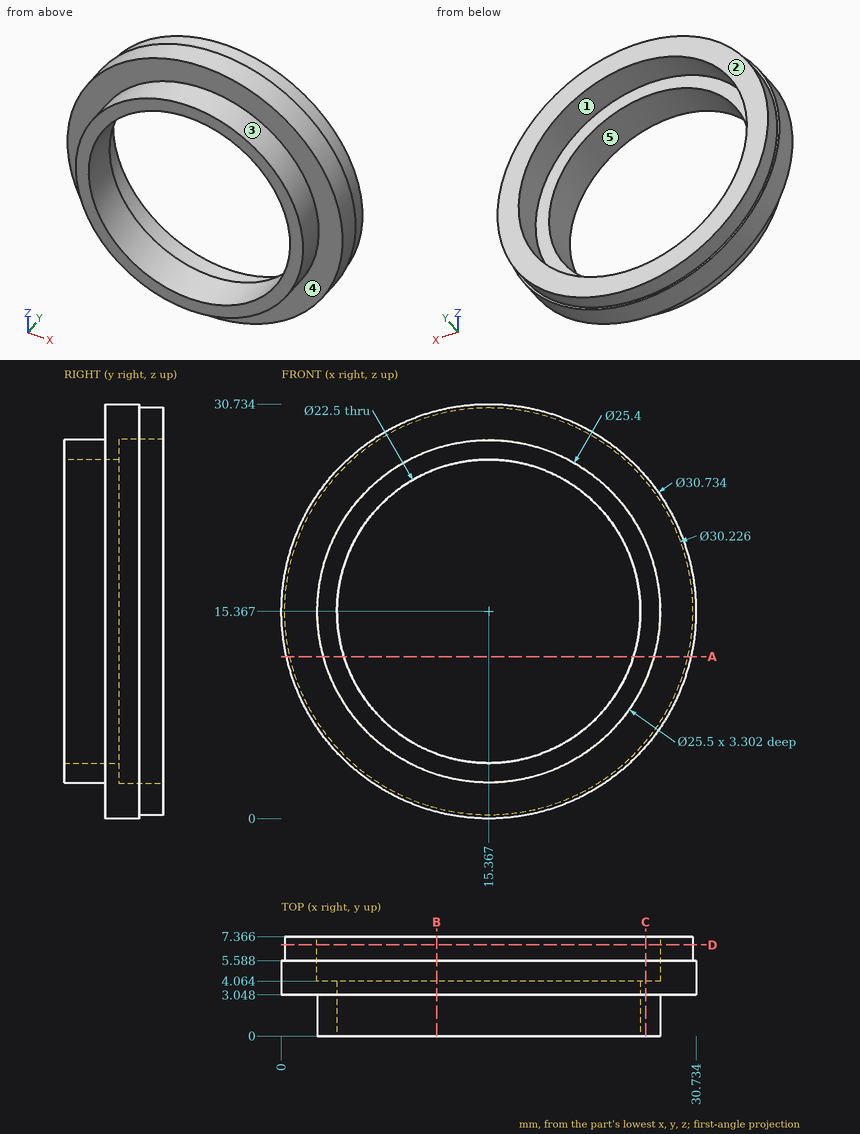
Geometry check sheet. Reference: drawing and pictorial views, mm from the part's lowest x, y, z. A direction names the side the tool comes from. Round coordinates to 2 decimals unless told otherwise and drop trailing zeros. Loops run counter-clockwise (first coordinate to the right, second up) from the corner with the lowest first, then second, coordinate; pieces in that order, holes last. Notation, with made-up numbers: M 47,50.5 L 80,50.5 A24 cw 80,73.5 Z; hole C -34.5,-15 d8. An arc over 180 degrees is marked long. One line per item, written item: value.
(1) Thickness scan on line 1 (X direction, y = 5.75, z = 15); line 2 (Y direction, x = 23, z = 2.5); line 3 (Z direction, x = 24.5, y = 5). Record the ranges inside material, lowest first.
Computed values:
line 1: x = 0.26 to 2.62, 28.11 to 30.48
line 2: y = 3.05 to 7.37
line 3: z = 3.01 to 6.47, 24.26 to 27.73
(2) Sectioned sample at D-D, the plane y = 6.75. Record the cut outline in (x, z).
Computed values:
outline: C 15.37,15.37 d30.23; hole C 15.37,15.37 d25.5
(3) Sectioned sample at A-A, the plane z = 12. Record the cut outline in (x, y), then the cut area to 3 significant figures.
Computed values:
outline: M 0.37,3.05 L 3.12,3.05 L 3.12,0 L 4.63,0 L 4.63,4.06 L 3.07,4.06 L 3.07,7.37 L 0.63,7.37 L 0.63,5.59 L 0.37,5.59 Z; M 26.1,0 L 27.61,0 L 27.61,3.05 L 30.36,3.05 L 30.36,5.59 L 30.1,5.59 L 30.1,7.37 L 27.66,7.37 L 27.66,4.06 L 26.1,4.06 Z
area: 34.7 mm^2
(4) Release check for a two-part mould opening along Z. For the marked faces 3, 4 and 5 record: +Z half, -Z half, draft (parallel to the pull), parting line (faces both ways), or undercut.
Computed values:
face 3: parting line
face 4: draft
face 5: undercut
(5) Depth check by flat-ended pin: pin 1 Ø1.5 at (y, z) = (4.5, 25.5) entering from +X; pin 2 Ø2 at (y, z) = (3.5, 26) entering from +X; pin 3 Ø1 at (x, y) = (24.5, 6.5) entering from -Z. Enter the tip coordinate at first touch or a pass-through.
Computed values:
pin 1: stops at x = 27.54
pin 2: stops at x = 27.34
pin 3: stops at z = 2.96
(6) Sectioned sample at C-C, the plane x = 27. Record the cut outline in (y, z), then the cut area to 3 significant figures.
Computed values:
outline: M 0,10.27 L 3.05,10.27 L 3.05,5.33 L 5.59,5.33 L 5.59,5.72 L 7.37,5.72 L 7.37,10.15 L 4.06,10.15 L 4.06,20.59 L 7.37,20.59 L 7.37,25.01 L 5.59,25.01 L 5.59,25.41 L 3.05,25.41 L 3.05,20.46 L 0,20.46 Z
area: 81.9 mm^2
(7) Access from +Z, -Z, +X, -X, +Y, -Y to the whole of each face (thin tool, end or side, straight path). Record for the marked faces 1 and 2.
Computed values:
face 1: +Y
face 2: +Z, -Z, +X, -X, +Y
(8) Sectioned sample at B-B, the plane x = 11.5. Record the cut outline in (y, z), then the cut area to 3 significant figures.
Computed values:
outline: M 0,3.27 L 3.05,3.27 L 3.05,0.49 L 5.59,0.49 L 5.59,0.76 L 7.37,0.76 L 7.37,3.22 L 4.06,3.22 L 4.06,4.8 L 0,4.8 Z; M 0,25.93 L 4.06,25.93 L 4.06,27.52 L 7.37,27.52 L 7.37,29.98 L 5.59,29.98 L 5.59,30.24 L 3.05,30.24 L 3.05,27.46 L 0,27.46 Z
area: 35.1 mm^2
